Print and shaded views of the part. All mm, measured from the part's lowest x, y and z. Coordinates: 2 decimals unless noted, no trailing zeros. Order: outer loops, then holes, each group sorted by start corner. A loop starts at its lowest first (then second) coordinate and runs counter-clockwise, first axis right, second up.
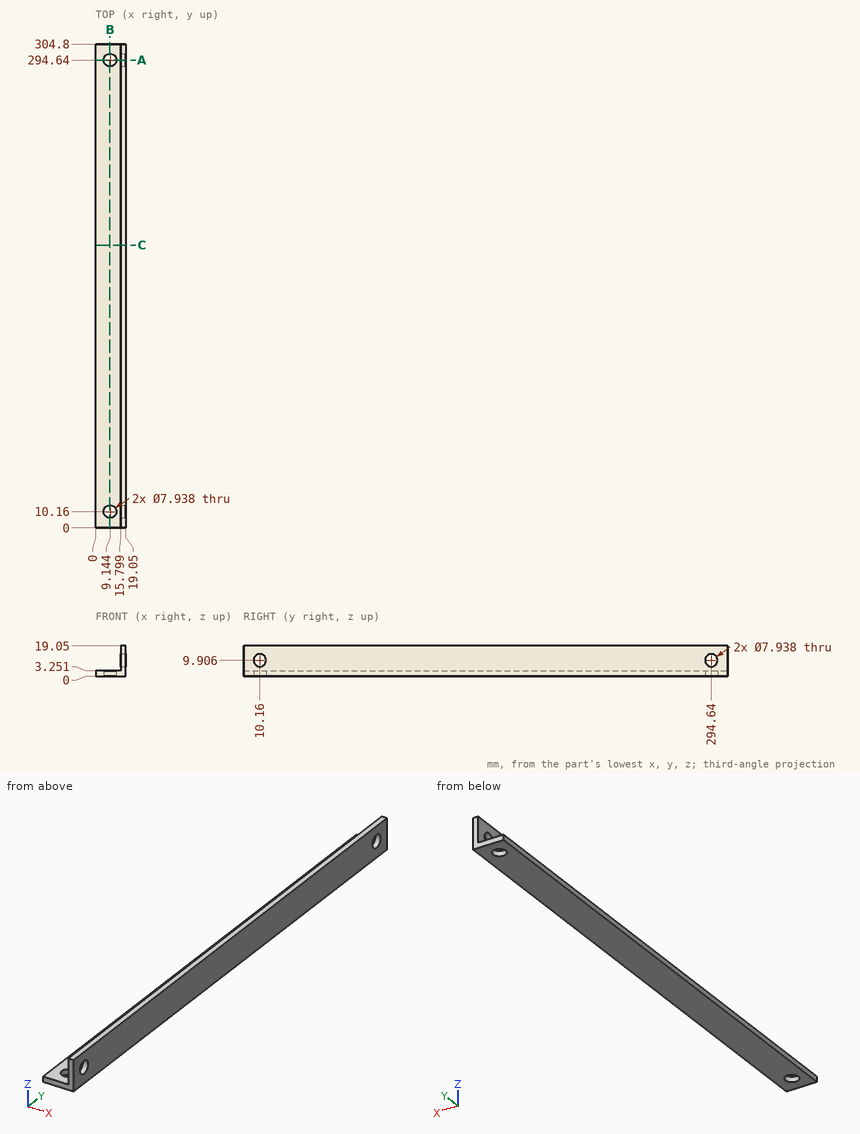
Q1. Cut at A-A, the plane y = 294.64. Count the separate pieces of the cut face and the enclosed holes in it.
Established:
separate pieces: 3
enclosed holes: 0
Q2. Probe line 1 (Y direction, x = 10, z = 2.75) (1 decimal); line 2 (X direction, y = 20.5, z = 17); line 3 (Z direction, x = 1.25, y = 55). List the from-to ranges inside material, lowest first.
Established:
line 1: y = 0 to 6.3, 14 to 290.8, 298.5 to 304.8
line 2: x = 15.8 to 19.05
line 3: z = 0 to 3.25
Q3. Cut at C-C, the plane y = 178. List the corners of the cut face in (x, z).
Established:
outline: (0, 0) - (19.05, 0) - (19.05, 19.05) - (15.8, 19.05) - (15.8, 3.25) - (0, 3.25) - close
Q4. Cut at B-B, the plane x = 9. List the corners of the cut face in (y, z).
Established:
outline: (0, 0) - (6.19, 0) - (6.19, 3.25) - (0, 3.25) - close; (14.13, 0) - (290.67, 0) - (290.67, 3.25) - (14.13, 3.25) - close; (298.61, 0) - (304.8, 0) - (304.8, 3.25) - (298.61, 3.25) - close
Q5. Drop flat-ended pins along their axis: P1, Ø10, axis at y = 38, z = 16, coming from the -X side; P2, Ø6.5, axis at x = 9.144, y = 294.64, coming from the +Z side; P3, Ø1, axis at x = 10, y = 91.5, coming from the +Z side. Give the stop position or say it passes through.
Established:
P1: stops at x = 15.8
P2: passes through
P3: stops at z = 3.25
